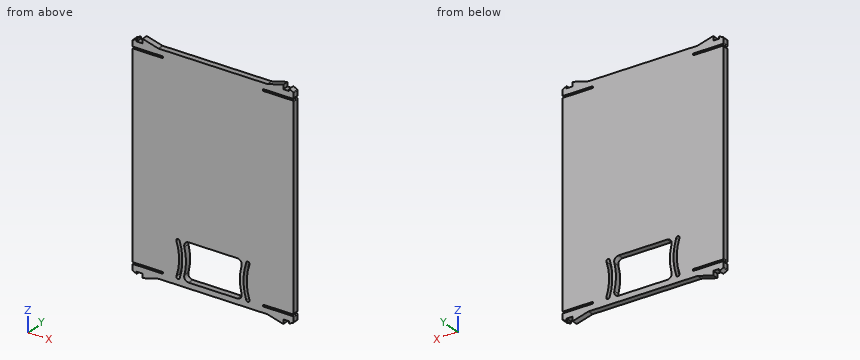
from build123d import *

# Parameters (mm, degrees)
PAD008_DEPTH = 2.8
FILLET001_R  = 0.4
POCKET_DEPTH = 2.801


with BuildPart() as part:
    # Sketch008 → Pad008 (new body)
    with BuildSketch(Plane(origin=(0, 20.1, 0), x_dir=(-1, 0, 0), z_dir=(0, 1, 0))):
        with BuildLine():
            Line((37.8, 63.2), (37.8, 60.4))
            Line((37.8, 60.4), (23.8, 60.4))
            ThreePointArc((23.8, 60.4), (23.4, 60), (23.8, 59.6))
            Line((23.8, 59.6), (37.8, 59.6))
            Line((37.8, 59.6), (37.8, -33.8))
            Line((37.8, -33.8), (23.8, -33.8))
            ThreePointArc((23.8, -33.8), (23.4, -34.2), (23.8, -34.6))
            Line((23.8, -34.6), (37.8, -34.6))
            Line((37.8, -34.6), (37.8, -37.4))
            Line((37.8, -37.4), (35.8, -38.4))
            Line((35.8, -38.4), (35.8, -37.4))
            Line((35.8, -37.4), (33, -37.4))
            Line((33, -39.4), (33, -37.4))
            Line((25.535898, -37.4), (33, -39.4))
            Line((-25.535898, -37.4), (25.535898, -37.4))
            Line((-33, -39.4), (-25.535898, -37.4))
            Line((-33, -37.4), (-33, -39.4))
            Line((-35.8, -37.4), (-33, -37.4))
            Line((-35.8, -38.4), (-35.8, -37.4))
            Line((-37.8, -37.4), (-35.8, -38.4))
            Line((-37.8, -37.4), (-37.8, -34.6))
            Line((-37.8, -34.6), (-23.8, -34.6))
            ThreePointArc((-23.8, -34.6), (-23.4, -34.2), (-23.8, -33.8))
            Line((-23.8, -33.8), (-37.8, -33.8))
            Line((-37.8, -33.8), (-37.8, 59.6))
            Line((-23.8, 59.6), (-37.8, 59.6))
            ThreePointArc((-23.8, 59.6), (-23.4, 60), (-23.8, 60.4))
            Line((-37.8, 60.4), (-23.8, 60.4))
            Line((-37.8, 60.4), (-37.8, 63.2))
            Line((-37.8, 63.2), (-35.8, 64.2))
            Line((-35.8, 64.2), (-35.8, 63.2))
            Line((-35.8, 63.2), (-33, 63.2))
            Line((-33, 65.2), (-33, 63.2))
            Line((-25.535898, 63.2), (-33, 65.2))
            Line((25.535898, 63.2), (-25.535898, 63.2))
            Line((33, 65.2), (25.535898, 63.2))
            Line((33, 63.2), (33, 65.2))
            Line((35.8, 63.2), (33, 63.2))
            Line((35.8, 64.2), (35.8, 63.2))
            Line((37.8, 63.2), (35.8, 64.2))
        make_face()
    extrude(amount=-PAD008_DEPTH)

    # Fillet001
    fillet001_edges = [part.edges().sort_by_distance(p)[0] for p in [
        (-37.8, 18.7, 59.6),
        (-37.8, 18.7, 60.4),
        (-37.8, 18.7, 63.2),
        (-25.535898, 18.7, 63.2),
        (25.535898, 18.7, 63.2),
        (37.8, 18.7, 63.2),
        (37.8, 18.7, 60.4),
        (37.8, 18.7, 59.6),
        (37.8, 18.7, -33.8),
        (37.8, 18.7, -34.6),
        (37.8, 18.7, -37.4),
        (25.535898, 18.7, -37.4),
        (-25.535898, 18.7, -37.4),
        (-37.8, 18.7, -37.4),
        (-37.8, 18.7, -33.8),
        (-37.8, 18.7, -34.6),
    ]]
    fillet(fillet001_edges, radius=FILLET001_R)

    # Sketch029 → Pocket (cut, through all)
    with BuildSketch(Plane(origin=(0, 20.1, 0), x_dir=(-1, 0, 0), z_dir=(0, 1, 0))):
        with BuildLine():
            Line((-11.39, -34.8), (11.39, -34.8))
            ThreePointArc((11.39, -34.8), (13.059932, -33.979739), (13.431495, -32.156708))
            ThreePointArc((13.431495, -19.843292), (12.640618, -26), (13.431495, -32.156708))
            ThreePointArc((13.431495, -19.843292), (13.059932, -18.020261), (11.39, -17.2))
            Line((11.39, -17.2), (-11.39, -17.2))
            ThreePointArc((-11.39, -17.2), (-13.059932, -18.020261), (-13.431495, -19.843292))
            ThreePointArc((-13.431495, -32.156708), (-12.640618, -26), (-13.431495, -19.843292))
            ThreePointArc((-13.431495, -32.156708), (-13.059932, -33.979739), (-11.39, -34.8))
        make_face()
        with BuildLine():
            ThreePointArc((-15.627473, -17.758024), (-16.639367, -17.239858), (-17.147686, -18.256734))
            ThreePointArc((-17.147686, -33.743266), (-15.87146, -26), (-17.147686, -18.256734))
            ThreePointArc((-17.147686, -33.743266), (-16.639367, -34.760142), (-15.627473, -34.241976))
            ThreePointArc((-15.627473, -34.241976), (-14.351104, -26), (-15.627473, -17.758024))
        make_face()
        with BuildLine():
            ThreePointArc((17.147686, -18.256734), (16.639367, -17.239858), (15.627473, -17.758024))
            ThreePointArc((15.627473, -17.758024), (14.351104, -26), (15.627473, -34.241976))
            ThreePointArc((15.627473, -34.241976), (16.639367, -34.760142), (17.147686, -33.743266))
            ThreePointArc((17.147686, -18.256734), (15.87146, -26), (17.147686, -33.743266))
        make_face()
    extrude(amount=-POCKET_DEPTH, mode=Mode.SUBTRACT)


solid = part.part
Here's how the part is built. I have some questions about the finished solid (model axes, mm). Give positions to 0.01 mm unless a question says otherwise; leave off trailing zeros. Loops run counter-clockwise (first coordinate to the right, second up) from the corner with the lowest first, then second, coordinate; pieces in that order, holes last. Notation, with made-up numbers: (11, 45.5) -> (64, 45.5) arc R25 cw to (64, 72.5) -> close; hole circle Ø2 at (14, -15.75). An arc over 180 degrees is marked (long way). One line per item, written item: value.
Q1. Suppose I cut it at B-B on z = -23. Please give me the cut outline in (x, y).
Answers follow:
outline: (-37.8, 17.3) -> (-16.06, 17.3) -> (-16.06, 20.1) -> (-37.8, 20.1) -> close; (-14.52, 17.3) -> (-12.83, 17.3) -> (-12.83, 20.1) -> (-14.52, 20.1) -> close; (12.83, 17.3) -> (14.52, 17.3) -> (14.52, 20.1) -> (12.83, 20.1) -> close; (16.06, 17.3) -> (37.8, 17.3) -> (37.8, 20.1) -> (16.06, 20.1) -> close
Q2. If I drill on line 1 along Z through (x, y) = (-34.5, 19.95); line 2 along Z through (x, y) = (-32, 19.4); line 3 along Z through (x, y) = (-3, 19.5), over which ranges is the centre line in solid material (lowest first)?
Answers follow:
line 1: -37.4 to -34.6, -33.8 to 59.6, 60.4 to 63.2
line 2: -39.13 to -34.6, -33.8 to 59.6, 60.4 to 64.93
line 3: -37.4 to -34.8, -17.2 to 63.2
Q3. I'm going to push flat-ended pins straight in: pin 1 Ø1.4 at (x, y) = (-30, 18.5) entering from +Z; pin 2 Ø1.4 at (x, y) = (-1.5, 18) entering from -Z; pin 3 Ø0.8 at (x, y) = (34, 19.5) entering from +Z. Where does each tip first touch, or does it pass through?
Answers follow:
pin 1: z = 64.58
pin 2: z = -37.4
pin 3: z = 63.2
Q4. Suppose I cut it at C-C on x = -30. Please give me the cut outline in (y, z), then the cut area to 3 significant figures.
Answers follow:
outline: (17.3, -38.6) -> (20.1, -38.6) -> (20.1, -34.6) -> (17.3, -34.6) -> close; (17.3, -33.8) -> (20.1, -33.8) -> (20.1, 59.6) -> (17.3, 59.6) -> close; (17.3, 60.4) -> (20.1, 60.4) -> (20.1, 64.4) -> (17.3, 64.4) -> close
area: 284 mm^2
Q5. Suppose I cut it at A-A on x = 7.5. Please give me the cut outline in (y, z).
Answers follow:
outline: (17.3, -37.4) -> (20.1, -37.4) -> (20.1, -34.8) -> (17.3, -34.8) -> close; (17.3, -17.2) -> (20.1, -17.2) -> (20.1, 63.2) -> (17.3, 63.2) -> close
Q6. Suppose I cut it at D-D on y = 18.6. State how many separate pieces and enclosed holes the cut face has, then the cut area to 3 significant figures.
Answers follow:
separate pieces: 1
enclosed holes: 3
area: 7,080 mm^2
